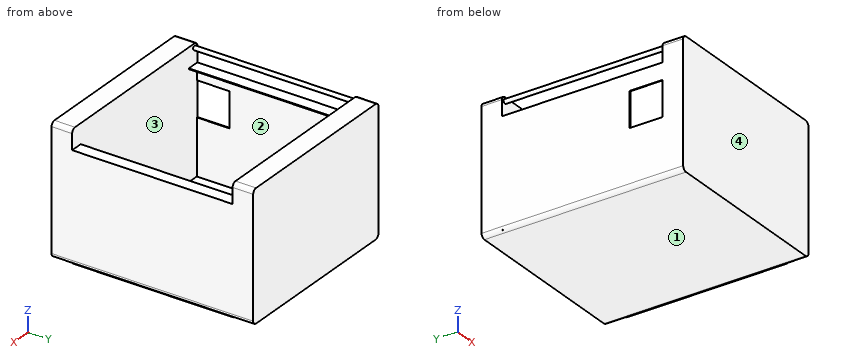
from build123d import *

# Parameters (mm, degrees)
SKETCH1_W           = 440
SKETCH1_H           = 310
BOSS_EXTRUDE1_DEPTH = 490
SHELL1_START        = -218
SHELL1_OUTLINE_W    = 390
SHELL1_OUTLINE_H    = 308
SHELL1_DEPTH        = 436
SKETCH3_W           = 440
SKETCH3_H           = 390
CUT_EXTRUDE1_DEPTH  = 50
SKETCH4_W           = 30
SKETCH4_H           = 390
BOSS_EXTRUDE2_DEPTH = 2
SKETCH5_W           = 30
SKETCH5_H           = 390
BOSS_EXTRUDE3_DEPTH = 2
SKETCH7_R           = 5
BOSS_EXTRUDE4_DEPTH = 440
FILLET1_R           = 10
FILLET2_R           = 10
CUT_EXTRUDE2_REACH  = 678.554
SKETCH8_W           = 85
SKETCH8_H           = 80


# Read off the part's stored shape, not the designer's step: Shell1
with BuildPart() as part:
    # Sketch1 → Boss-Extrude1 (new body)
    with BuildSketch(Plane(origin=(0, 0, 0), x_dir=(1, 0, 0), z_dir=(0, 1, 0))):
        Rectangle(SKETCH1_W, SKETCH1_H)
    extrude(amount=BOSS_EXTRUDE1_DEPTH)

    # Shell1 outline → Shell1 (cut)
    with BuildSketch(Plane.YZ.offset(SHELL1_START)):
        with Locations((245, 1)):
            Rectangle(SHELL1_OUTLINE_W, SHELL1_OUTLINE_H)
    extrude(amount=SHELL1_DEPTH, mode=Mode.SUBTRACT)

    # Sketch3 → Cut-Extrude1 (cut)
    with BuildSketch(Plane.XY.offset(155)):
        with Locations((0, 245)):
            Rectangle(SKETCH3_W, SKETCH3_H)
    extrude(amount=-CUT_EXTRUDE1_DEPTH, mode=Mode.SUBTRACT)

    # Sketch4 → Boss-Extrude2 (add)
    with BuildSketch(Plane.XY.offset(105)):
        with Locations((-205, 245)):
            Rectangle(SKETCH4_W, SKETCH4_H)
    extrude(amount=BOSS_EXTRUDE2_DEPTH)

    # Sketch5 → Boss-Extrude3 (add)
    with BuildSketch(Plane.XY.offset(105)):
        with Locations((205, 245)):
            Rectangle(SKETCH5_W, SKETCH5_H)
    extrude(amount=BOSS_EXTRUDE3_DEPTH)

    # Sketch7 → Boss-Extrude4 (add)
    with BuildSketch(Plane(origin=(0, 50, 0), x_dir=(1, 0, 0), z_dir=(0, 1, 0))):
        with Locations(Location((-210, -145, 0), (0, 0, 90))):
            Circle(SKETCH7_R)
    extrude(amount=BOSS_EXTRUDE4_DEPTH)

    # Fillet1
    fillet1_edges = [part.edges().sort_by_distance(p)[0] for p in [
        (-220, 25, 155),
        (220, 25, 155),
        (220, 465, 155),
        (-220, 465, 155),
    ]]
    fillet(fillet1_edges, radius=FILLET1_R)

    # Fillet2
    fillet2_edges = [part.edges().sort_by_distance(p)[0] for p in [
        (-220, 245, -155),
        (220, 245, -155),
    ]]
    fillet(fillet2_edges, radius=FILLET2_R)

    # Sketch8 → Cut-Extrude2 (cut, up to next)
    with BuildSketch(Plane.ZY.offset(220), mode=Mode.PRIVATE) as cut_extrude2_sk1:
        with Locations((24.5, 90)):
            Rectangle(SKETCH8_W, SKETCH8_H)
    cut_extrude2_tool1 = extrude(cut_extrude2_sk1.sketch, amount=-CUT_EXTRUDE2_REACH, mode=Mode.PRIVATE) & part.part
    add(cut_extrude2_tool1.solids().sort_by_distance((-220, 90, 24.5))[0], mode=Mode.SUBTRACT)


solid = part.part
The model under review builds one solid part; all positions refer to its coordinate system, in mm. Face numbers are marked on the shaded views. Give positions to 0.01 mm unless a question says otherwise; leave off trailing zeros. Write each loop counter-clockwise with the first axis right and the second up, starting at its lowest first coordinate (ties: lowest second). Pieces come first, ordered by that corner, then holes.
1. Draft analysis for pull direction Y (two halves, no side actions). For the marked faces 1, 2, 3 and 4, state which applies: +Y half, -Y half, draft (parallel to the pull), parting line (faces both ways), or undercut.
2. Wall thickness on L1, parallel to Y at x = 186.5, z = -96.5; L2, parallel to Z at x = -190.5, y = 83; L3, parallel to X at y = 407.5, z = -111: over which ranges is each line inside the solid? List them lowest first.
3. Add section B-B, the plane z = 117.5. Write out the cut boundary in (x, y).
4. For P1, Ø6, axis at x = -26.5, y = 386.5, coming from the +Z side; P2, Ø1.6, axis at x = -219, y = 73.5, coming from the +Z side; P3, Ø2, axis at x = -219.5, y = 77.5, coming from the -Z side, all flat-tipped, find the tip position at first contact; note any pin that passes through.
5. Add section D-D, the plane z = 82. Write out the cut boundary in (x, y), plus the area to 3 significant figures.
Worked answers:
1. face 1: draft
1. face 2: undercut
1. face 3: undercut
1. face 4: -Y half
2. L1: y = 0 to 50, 440 to 490
2. L2: z = -155 to -153, 105 to 107
2. L3: x = -220 to -218, 218 to 220
3. outline: (-220, 0) - (220, 0) - (220, 50) - (-220, 50) - close; (-220, 440) - (220, 440) - (220, 490) - (-220, 490) - close
4. P1: stops at z = -153
4. P2: stops at z = 107
4. P3: stops at z = -150.27
5. outline: (-220, 0) - (220, 0) - (220, 490) - (-220, 490) - close; hole (-218, 50) - (218, 50) - (218, 440) - (-218, 440) - close
5. area: 45,600 mm2
